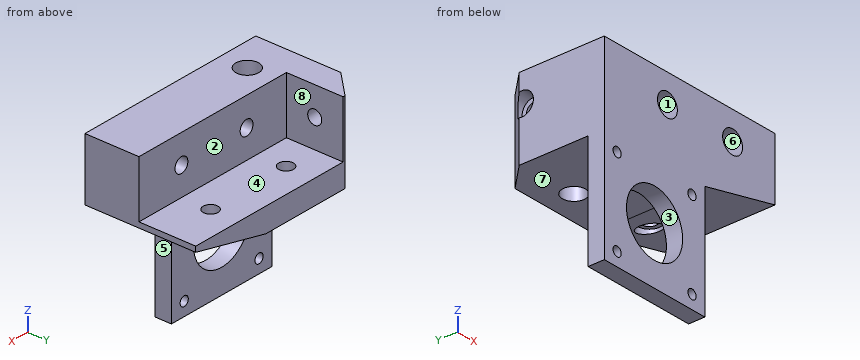
from build123d import *

# Parameters (mm, degrees)
SKETCH_1_R          = 12
SKETCH_1_R_2        = 1.75
EXTRUDE_1_DEPTH     = 6
EXTRUDE_2_DEPTH     = 35
SKETCH_3_W          = 63
SKETCH_3_H          = 21
CUT_EXTRUDE_1_DEPTH = 21
SKETCH_4_R          = 2.6
CUT_EXTRUDE_2_DEPTH = 87.609201921
CHAMFER_1_SIZE      = 9.5
CHAMFER_1_SIZE_2    = 9.174043361
CUT_EXTRUDE_START   = -10
SKETCH_5_R          = 4.25
CUT_EXTRUDE_3_DEPTH = 5
SKETCH_6_R          = 2.75
CUT_EXTRUDE_4_DEPTH = 78.360370477
CUT_EXTRUDE_START_2 = -4
SKETCH_7_R          = 4.25
CUT_EXTRUDE_5_DEPTH = 5
SKETCH_8_R          = 2.75
CUT_EXTRUDE_6_DEPTH = 64.20427816
SKETCH_10_R         = 4.25
CUT_EXTRUDE_7_DEPTH = 15.5
SKETCH_11_R         = 4.25
CUT_EXTRUDE_8_DEPTH = 20


with BuildPart() as part:
    # Эскиз1 → Бобышка-Вытянуть1 (new body)
    with BuildSketch(Plane(origin=(0, 0, 0), x_dir=(1, 0, 0), z_dir=(0, 1, 0))):
        Polygon((-31.737099952, -43.025037564), (41.262900048, -43.025037564), (41.262900048, -20.025037564), (11.262900048, -13.109402144), (11.262900048, 28.974962436), (-31.737099952, 28.974962436), align=None)
        with Locations(Location((-10.237099952, 7.974962436, 0), (0, 0, 270))):
            Circle(SKETCH_1_R, mode=Mode.SUBTRACT)
        with Locations(Location((-26.237099952, 23.974962436, 0), (0, 0, 270))):
            Circle(SKETCH_1_R_2, mode=Mode.SUBTRACT)
        with Locations(Location((5.762900048, 23.974962436, 0), (0, 0, 270))):
            Circle(SKETCH_1_R_2, mode=Mode.SUBTRACT)
        with Locations(Location((5.762900048, -8.025037564, 0), (0, 0, 270))):
            Circle(SKETCH_1_R_2, mode=Mode.SUBTRACT)
        with Locations(Location((-26.237099952, -8.025037564, 0), (0, 0, 270))):
            Circle(SKETCH_1_R_2, mode=Mode.SUBTRACT)
    extrude(amount=EXTRUDE_1_DEPTH)

    # Эскиз2 → Бобышка-Вытянуть2 (add)
    with BuildSketch(Plane(origin=(0, 6, 0), x_dir=(1, 0, 0), z_dir=(0, 1, 0))):
        Polygon((41.262900048, -20.025037564), (11.262900048, -13.109402144), (-31.737099952, -13.109402144), (-31.737099952, -43.025037564), (41.262900048, -43.025037564), align=None)
    extrude(amount=EXTRUDE_2_DEPTH)

    # Эскиз3 → Вырез-Вытянуть1 (cut)
    with BuildSketch(Plane(origin=(0, 41, 0), x_dir=(1, 0, 0), z_dir=(0, 1, 0))):
        with Locations((9.762900048, -32.525037564)):
            Rectangle(SKETCH_3_W, SKETCH_3_H)
    extrude(amount=-CUT_EXTRUDE_1_DEPTH, mode=Mode.SUBTRACT)

    # Эскиз4 → Вырез-Вытянуть2 (cut, through all)
    with BuildSketch(Plane(origin=(-21.737099952, 0, 0), x_dir=(0, 0, -1), z_dir=(1, 0, 0))):
        with Locations((-32.525037564, 30.5)):
            Circle(SKETCH_4_R)
    extrude(amount=-CUT_EXTRUDE_2_DEPTH, mode=Mode.SUBTRACT)

    # Фаска1
    # the kernel refuses this chamfer: 9.5, 9.174043361 mm, written as the material it takes off along each edge
    with BuildSketch(Plane(origin=(-31.737099952, 41, -11.332881065), x_dir=(-0.026999337430198715, -0.9996354514413394, 0), z_dir=(0, 0, 1))) as chamfer_1_piece_1:
        Polygon((CHAMFER_1_SIZE * 0.999635451441, CHAMFER_1_SIZE * 0.0269993374302), (-CHAMFER_1_SIZE_2 * 0.0269993374292, CHAMFER_1_SIZE_2 * 0.999635451405), (0, 0), align=None)
    extrude(amount=78.800201839, mode=Mode.SUBTRACT)

    # Эскиз5 → Вырез-Вытянуть3 (cut)
    with BuildSketch(Plane(origin=(-21.737099952, 0, 0), x_dir=(0, 0, -1), z_dir=(1, 0, 0)).offset(CUT_EXTRUDE_START)):
        with Locations(Location((-32.525037564, 30.5, 0), (0, 0, 166.391039369))):
            Circle(SKETCH_5_R)
    extrude(amount=CUT_EXTRUDE_3_DEPTH, mode=Mode.SUBTRACT)

    # Эскиз6 → Вырез-Вытянуть4 (cut, through all)
    with BuildSketch(Plane.XY.offset(22.025037564)):
        with Locations((-9.495708976, 30.5)):
            Circle(SKETCH_6_R)
        with Locations((22.785725254, 30.5)):
            Circle(SKETCH_6_R)
    extrude(amount=-CUT_EXTRUDE_4_DEPTH, mode=Mode.SUBTRACT)

    # Эскиз7 → Вырез-Вытянуть5 (cut)
    with BuildSketch(Plane.XY.offset(22.025037564).offset(CUT_EXTRUDE_START_2)):
        with Locations((-9.495708976, 30.5)):
            Circle(SKETCH_7_R)
        with Locations((22.785725254, 30.5)):
            Circle(SKETCH_7_R)
    extrude(amount=-CUT_EXTRUDE_5_DEPTH, mode=Mode.SUBTRACT)

    # Эскиз8 → Вырез-Вытянуть6 (cut, through all)
    with BuildSketch(Plane(origin=(0, 20, 0), x_dir=(1, 0, 0), z_dir=(0, 1, 0))):
        with Locations(Location((-4.737013791, -32.525037564, 0), (0, 0, 270))):
            Circle(SKETCH_8_R)
        with Locations(Location((23.126402015, -32.525037564, 0), (0, 0, 270))):
            Circle(SKETCH_8_R)
    extrude(amount=-CUT_EXTRUDE_6_DEPTH, mode=Mode.SUBTRACT)

    # Эскиз10 → Вырез-Вытянуть7 (cut)
    with BuildSketch(Plane.XZ):
        with Locations(Location((23.126402015, 32.525037564, 0), (0, 0, 270))):
            Circle(SKETCH_10_R)
        with Locations(Location((-4.737013791, 32.525037564, 0), (0, 0, 270))):
            Circle(SKETCH_10_R)
    extrude(amount=-CUT_EXTRUDE_7_DEPTH, mode=Mode.SUBTRACT)

    # Эскиз11 → Вырез-Вытянуть8 (cut)
    with BuildSketch(Plane.XY.offset(43.025037564)):
        with Locations((-16.587099952, 10)):
            Circle(SKETCH_11_R)
    extrude(amount=-CUT_EXTRUDE_8_DEPTH, mode=Mode.SUBTRACT)


solid = part.part
CAD build for the part. Positions are in the model's coordinates, mm. Face numbers are marked on the shaded views. A direction names the side the tool comes from. Round coordinates to 2 decimals unless told otherwise and drop trailing zeros. Write each loop counter-clockwise with the first axis right and the second up, starting at its lowest first coordinate (ties: lowest second). Pieces come first, ordered by that corner, then holes.
(1) Slice it at B-B, the plane z = 2. Write the cut outline in (x, y), and give its area (3 significant figures).
(2) Slice it at A-A, the plane y = 30.5. Count the separate pieces of the cut face and the enclosed holes in it, and give its area (3 significant figures).
(3) Mould opens along Z. For the marked faces 1, 2, 3 and 4 say: pulls with the +Z half, pulls with the -Z half, needs draft (parallel to the pull), parting line crosses it, or undercut.
(4) Probe line 1 along Y through (x, z) = (-16.5, 29); line 2 along Y through (x, z) = (28, 24); line 3 along Z through (x, y) = (7, 33). List the from-to ranges inside material, lowest first.
(5) Drop flat-ended pins along their axis: P1, Ø6.5, axis at x = 6, z = 28, coming from the +Y side; P2, Ø4, axis at x = -5, z = 34, coming from the -Y side; P3, Ø7.5, axis at x = -9.5, y = 30.5, coming from the +Z side. Give the stop position or say it passes through.
(6) Slice it at C-C, the plane z = 19. Write the cut outline in (x, y), and give its area (3 significant figures).
(7) 3-axis set-ups, long thin cutter, end or side, ignore diameter. For the marked faces 5, 6, 7 and 8: which of +Z, -Z, +X, -X, +Y, -Y reach the whole face in a straight line?
(8) Slice it at D-D, the plane y = 10. Write the cut outline in (x, z), and give its area (3 significant figures).
From the geometry:
1. outline: (-31.74, 0) - (-16.91, 0) - (-16.91, 6) - (-31.74, 6) - close; (-3.57, 0) - (11.26, 0) - (11.26, 6) - (-3.57, 6) - close
1. area: 178 mm2
2. separate pieces: 4
2. enclosed holes: 0
2. area: 584 mm2
3. face 1: undercut
3. face 2: needs draft
3. face 3: undercut
3. face 4: pulls with the +Z half
4. line 1: y = 0 to 5.75, 14.25 to 20
4. line 2: y = 0 to 20
4. line 3: z = 13.11 to 22.03
5. P1: stops at y = 20
5. P2: stops at y = 15.5
5. P3: stops at z = 22.03
6. outline: (-31.74, 0) - (36.82, 0) - (36.82, 41) - (-22.56, 41) - (-31.74, 31.5) - close; hole circle Ø5.5 at (-9.5, 30.5); hole circle Ø5.5 at (22.79, 30.5)
6. area: 2,720 mm2
7. face 5: -Z, +X, +Y, -Y
7. face 6: -Y
7. face 7: -Z, +X, -X, +Y
7. face 8: +Z, +X, +Y
8. outline: (-31.74, 13.11) - (11.26, 13.11) - (41.26, 20.03) - (41.26, 43.03) - (-12.34, 43.03) - (-12.34, 23.03) - (-20.84, 23.03) - (-20.84, 43.03) - (-31.74, 43.03) - close; hole circle Ø8.5 at (-4.74, 32.53); hole circle Ø8.5 at (23.13, 32.53)
8. area: 1,800 mm2
